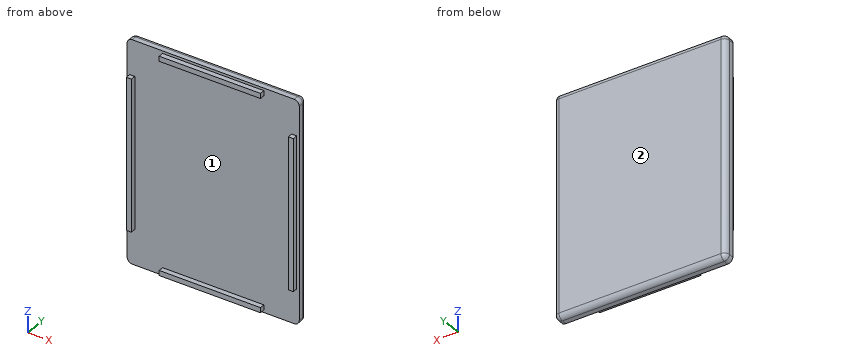
Autodesk Inventor part; units mm, degrees
ref_plane "YZ Plane" through (0, 0, 0) normal (1, 0, 0) x (0, 1, 0)
ref_plane "XZ Plane" through (0, 0, 0) normal (0, 1, 0) x (-1, 0, 0)
ref_plane "XY Plane" through (0, 0, 0) normal (0, 0, 1) x (1, 0, 0)
sketch "Sketch4" plane through (0, 0, 0) normal (0, 1, 0) x (-1, 0, 0)
  line L0 (17, 22) -> (-17, 22)
  line L1 (-17, 22) -> (-17, -22)
  line L2 (-17, -22) -> (17, -22)
  line L3 (17, -22) -> (17, 22)
  line L4 (17, 22) -> (-17, -22) construction
  line L5 (-17, 22) -> (17, -22) construction
  point P0 (0, 0)
  dimension "d52" = 34
  dimension "d53" = 44
extrude "Extrusion5" add sketch "Sketch4" along normal blind 2
sketch "Sketch6" plane through (0, 0, 0) normal (0, -1, 0) x (1, 0, 0)
  line L0 (-16.5, -15) -> (-15.5, -15)
  line L1 (-15.5, -15) -> (-15.5, 5)
  line L2 (-15.5, 5) -> (-16.5, 5)
  line L3 (-16.5, 5) -> (-16.5, -15)
  line L4 (-15.5, -5) -> (-16.5, -5)
  line L5 (-16.5, -5) -> (-16.5, 15)
  line L6 (-16.5, 15) -> (-15.5, 15)
  line L7 (-15.5, 15) -> (-15.5, -5)
  line L8 (-10, 21.5) -> (10, 21.5)
  line L9 (10, 21.5) -> (10, 20.5)
  line L10 (10, 20.5) -> (-10, 20.5)
  line L11 (-10, 20.5) -> (-10, 21.5)
  line L12 (10, 21.5) -> (-10, 21.5)
  line L13 (-10, 21.5) -> (-10, 20.5)
  line L14 (-10, 20.5) -> (10, 20.5)
  line L15 (10, 20.5) -> (10, 21.5)
  line L16 (15.5, 15) -> (16.5, 15)
  line L17 (16.5, 15) -> (16.5, -5)
  line L18 (16.5, -5) -> (15.5, -5)
  line L19 (15.5, -5) -> (15.5, 15)
  line L20 (15.5, -15) -> (16.5, -15)
  line L21 (16.5, -15) -> (16.5, 5)
  line L22 (16.5, 5) -> (15.5, 5)
  line L23 (15.5, 5) -> (15.5, -15)
  line L24 (10, -20.5) -> (-10, -20.5)
  line L25 (-10, -20.5) -> (-10, -21.5)
  line L26 (-10, -21.5) -> (10, -21.5)
  line L27 (10, -21.5) -> (10, -20.5)
  line L28 (-10, -20.5) -> (10, -20.5)
  line L29 (10, -20.5) -> (10, -21.5)
  line L30 (10, -21.5) -> (-10, -21.5)
  line L31 (-10, -21.5) -> (-10, -20.5)
  line L32 (-17, 22) -> (-17, -22)
  line L33 (17, 22) -> (-17, 22)
  line L34 (17, -22) -> (17, 22)
  line L35 (-17, -22) -> (17, -22)
  line L36 (17, 22) -> (17, -22)
  line L37 (-17, -22) -> (-17, 22)
  line L38 (-17, 22) -> (17, 22)
  line L39 (17, -22) -> (-17, -22)
  point P0 (0, 0)
  point P1 (-16, 15)
  point P2 (-16, -5)
  point P3 (16, 15)
  point P4 (16, -15)
  point P5 (-10, -21)
  point P6 (-16, -15)
  dimension "d123" = 1
  dimension "d124" = 20
  dimension "d119" = 1
  dimension "d118" = 20
  dimension "d116" = 20
  dimension "d117" = 1
  dimension "d112" = 20
  dimension "d113" = 1
  dimension "d108" = 1
  dimension "d109" = 20
  dimension "d104" = 1
  dimension "d105" = 20
  dimension "d101" = 20
  dimension "d102" = 1
  dimension "d97" = 20
  dimension "d98" = 1
  dimension "d114" = 7
  dimension "d115" = 0.5
  dimension "d111" = 0.5
  dimension "d110" = 7
  dimension "d107" = 7
  dimension "d106" = 0.5
  dimension "d103" = 0.5
  dimension "d95" = 7
  dimension "d99" = 7
  dimension "d100" = 0.5
  dimension "d96" = 0.5
  dimension "d94" = 7
  dimension "d93" = 7
  dimension "d122" = 0.5
  dimension "d120" = 7
  dimension "d121" = 0.5
  dimension "d133" = 0
  dimension "d134" = 0
  dimension "d135" = 0
  dimension "d136" = 0
extrude "Extrusion7" add sketch "Sketch6" along normal blind 1 contours L3 L4 L1 L0 | L3 L2 L1 L4 | L5 L6 L7 L2 | L8 L9 L10 L11 | L16 L17 L22 L19 | L22 L17 L18 L19 | L18 L21 L20 L23 | L27 L26 L25 L24
fillet "Fillet9" radius 1 1 edges at (17, 1, -22)
fillet "Fillet10" radius 1 1 edges at (-17, 1, -22)
fillet "Fillet11" radius 1 1 edges at (-17, 1, 22)
fillet "Fillet12" radius 1 1 edges at (17, 1, 22)
fillet "Fillet13" radius 1 8 edges at (-16.7071, 2, -21.7071) (-17, 2, 0) (-16.7071, 2, 21.7071) (0, 2, 22) (16.7071, 2, 21.7071) (17, 2, 0) (16.7071, 2, -21.7071) (0, 2, -22)
properties part number "block_main" material "PC/ABS Plastic"
Verification items for the finished model (mm, model axes). Face numbers are marked on the shaded views. Round coordinates to 2 decimals unless told otherwise and drop trailing zeros. Write each loop counter-clockwise with the first axis right and the second up, starting at its lowest first coordinate (ties: lowest second). Pieces come first, ordered by that corner, then holes.
(1) Material ranges on line 1 (X direction, y = -0.05, z = -13); line 2 (Z direction, x = -9, y = -0.55); line 3 (Y direction, x = -14, z = -15), recorded low to high.
Returned:
line 1: x = -16.5 to -15.5, 15.5 to 16.5
line 2: z = -21.5 to -20.5, 20.5 to 21.5
line 3: y = 0 to 2
(2) Section check B-B (z = -6.5). Enter the section's corners in (x, y).
Returned:
outline: (-17, 0) - (-16.5, 0) - (-16.5, -1) - (-15.5, -1) - (-15.5, 0) - (15.5, 0) - (15.5, -1) - (16.5, -1) - (16.5, 0) - (17, 0) - (17, 1) arc R1 ccw to (16, 2) - (-16, 2) arc R1 ccw to (-17, 1) - close
(3) Section check D-D (z = -17.5). Enter the section's corners in (x, y), plus the area to 3 significant figures.
Returned:
outline: (-17, 0) - (17, 0) - (17, 1) arc R1 ccw to (16, 2) - (-16, 2) arc R1 ccw to (-17, 1) - close
area: 67.6 mm2
(4) Section check C-C (x = 6). Enter the section's corners in (y, z), plus the area to 3 significant figures.
Returned:
outline: (-1, -21.5) - (0, -21.5) - (0, -22) - (1, -22) arc R1 ccw to (2, -21) - (2, 21) arc R1 ccw to (1, 22) - (0, 22) - (0, 21.5) - (-1, 21.5) - (-1, 20.5) - (0, 20.5) - (0, -20.5) - (-1, -20.5) - close
area: 89.6 mm2
(5) Depth check by flat-ended pin: pin 1 Ø0.5 at (x, y) = (3.5, -0.5) entering from +Z; pin 2 Ø0.8 at (y, z) = (-0.5, 5.5) entering from +X; pin 3 Ø0.5 at (y, z) = (-0.5, 21) entering from -X. Enter the tip coordinate at first touch or a pass-through.
Returned:
pin 1: stops at z = 21.5
pin 2: stops at x = 16.5
pin 3: stops at x = -10
(6) Mould release check, pull along Z, two halves, no side actions. Record for the marked faces 1 and 2: pulls with the +Z half, pulls with the -Z half, needs draft (parallel to the pull), parting line crosses it, or undercut.
Returned:
face 1: undercut
face 2: needs draft
(7) Section check A-A (y = -0.55). Enter the section's corners in (x, z), plus the area to 3 significant figures.
Returned:
outline: (-16.5, -15) - (-15.5, -15) - (-15.5, 15) - (-16.5, 15) - close; (-10, -21.5) - (10, -21.5) - (10, -20.5) - (-10, -20.5) - close; (-10, 20.5) - (10, 20.5) - (10, 21.5) - (-10, 21.5) - close; (15.5, -15) - (16.5, -15) - (16.5, 15) - (15.5, 15) - close
area: 100 mm2
